from build123d import *

# Parameters (mm, degrees)
SKETCH1_W            = 12.7
SKETCH1_H            = 104.775
BOSS_EXTRUDE1_DEPTH  = 6.35
M3_CLEARANCE_HOLE1_D = 3.4
FILLET1_R            = 6.35


with BuildPart() as part:
    # Sketch1 → Boss-Extrude1 (new body)
    with BuildSketch(Plane(origin=(0, 0, 0), x_dir=(0, 0, -1), z_dir=(1, 0, 0))):
        with Locations((-37.097368421, 4.528552632)):
            Rectangle(SKETCH1_W, SKETCH1_H)
    extrude(amount=BOSS_EXTRUDE1_DEPTH)

    # M3 Clearance Hole1 (through all)
    with Locations(Plane(origin=(0, 0, 30.747368421), x_dir=(-1, 0, 0), z_dir=(0, 0, -1))):
        with Locations((-3.175, -25.996447368), (-3.175, 4.528552632), (-3.175, 35.053552632)):
            Hole(M3_CLEARANCE_HOLE1_D / 2)

    # Fillet1
    fillet1_edges = [part.edges().sort_by_distance(p)[0] for p in [
        (3.175, -47.858947368, 43.447368421),
        (3.175, 56.916052632, 43.447368421),
    ]]
    fillet(fillet1_edges, radius=FILLET1_R)


solid = part.part
Can you work these out from the model? Positions are in its coordinate system, mm. Give positions to 0.01 mm unless a question says otherwise; leave off trailing zeros. Loops run counter-clockwise (first coordinate to the right, second up) from the corner with the lowest first, then second, coordinate; pieces in that order, holes last. Notation, with made-up numbers: (-37.5, -18) -> (-23.5, -18) arc R15 cw to (-23.5, -2) -> close; hole circle Ø11 at (70.5, 36). An arc over 180 degrees is marked (long way). Use one line per item in the form item = value.
1) I need wall thicknesses on line 1 along Y through (x, z) = (3, 37); line 2 along Y through (x, z) = (4, 41); line 3 along Y through (x, z) = (5, 42.25). Which ranges of each line are inside material? Lowest first, please.
Answers:
line_1 = -47.86 to -27.69, -24.31 to 2.84, 6.22 to 33.36, 36.74 to 56.92
line_2 = -46.52 to -27.48, -24.51 to 3.04, 6.01 to 33.57, 36.54 to 55.58
line_3 = -45.22 to 54.28
2) If we section it at C-C (z = 32.75): Please give me the cut outline in (x, y) (3 decimals).
Answers:
outline = (0, -47.859) -> (6.35, -47.859) -> (6.35, 56.916) -> (0, 56.916) -> close; hole circle Ø3.4 at (3.175, -25.996); hole circle Ø3.4 at (3.175, 4.529); hole circle Ø3.4 at (3.175, 35.054)
3) If we section it at A-A (x = 3.25): Please give me the cut outline in (y, z), plus the area to 3 significant figures.
Answers:
outline = (-47.86, 30.75) -> (-27.69, 30.75) -> (-27.69, 43.45) -> (-41.51, 43.45) arc R6.35 ccw to (-47.86, 37.1) -> close; (-24.3, 30.75) -> (2.83, 30.75) -> (2.83, 43.45) -> (-24.3, 43.45) -> close; (6.23, 30.75) -> (33.36, 30.75) -> (33.36, 43.45) -> (6.23, 43.45) -> close; (36.75, 30.75) -> (56.92, 30.75) -> (56.92, 37.1) arc R6.35 ccw to (50.57, 43.45) -> (36.75, 43.45) -> close
area = 1,180 mm²
4) We'd pull the mould along Y, two halves only. Please class faces 1 (the face through (5, 4, 30.747)), 2 (the face through (2.95, -24.31, 37.19)), 3 (the face through (3, -47.859, 34)): released by +Y, released by -Y, zero draft, split by the parting line, or undercut.
Answers:
face_1 = zero draft
face_2 = undercut
face_3 = released by -Y
5) If we section it at B-B (z = 38.75): Please give me the cut outline in (x, y) (3 decimals).
Answers:
outline = (0, -47.64) -> (6.35, -47.64) -> (6.35, 56.697) -> (0, 56.697) -> close; hole circle Ø3.4 at (3.175, -25.996); hole circle Ø3.4 at (3.175, 4.529); hole circle Ø3.4 at (3.175, 35.054)
6) Will this pin go through, and if not, where does the flat tip stop? pin 1 (2.5 mm diameter, centred on x = 3.18, y = -26, fed in from -Z).
Answers:
pin_1 = through
